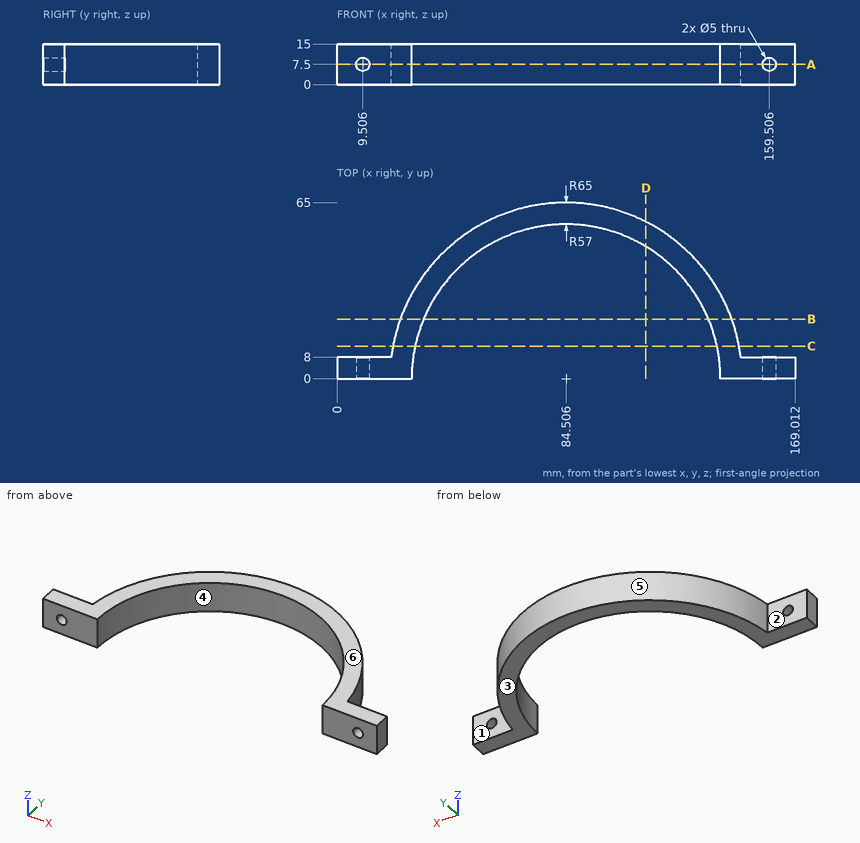
The drawing under review shows one solid part. Ordinate dimensions are in mm from its lowest x, y, z. A direction names the side the tool comes from. Round coordinates to 2 decimals unless told otherwise and drop trailing zeros. Write each loop counter-clockwise with the first axis right and the second up, starting at its lowest first coordinate (ties: lowest second). Pieces come first, ordered by that corner, then holes. Notation, with made-up numbers: (81.25, 50) - (93.25, 50) arc R21 ccw to (93.25, 54) - close; hole circle Ø7 at (-33.5, 86). An arc over 180 degrees is marked (long way). Use one line per item in the form item = value.
Q1. For line 1 (X direction, y = 47, z = 8.75) (1 decimal); line 2 (Y direction, x = 14, z = 10); line 3 (Y direction, x = 135, z = 5) (1 decimal), list the stretches that pass through material, from the lowest coordinate up. Write a range as [from, to].
Answer key:
line_1 = [39.6, 52.3], [116.8, 129.4]
line_2 = [0, 8]
line_3 = [26.4, 40.9]
Q2. Consider section A-A (z = 7.5). State the section outline as (x, y) points.
Answer key:
outline = (0, 0) - (7.01, 0) - (7.01, 8) - (0, 8) - close; (12.01, 0) - (27.51, 0) arc R57 cw to (141.51, 0) - (157.01, 0) - (157.01, 8) - (149.01, 8) arc R65 ccw to (20, 8) - (12.01, 8) - close; (162.01, 0) - (169.01, 0) - (169.01, 8) - (162.01, 8) - close
Q3. Insertion check: pin 1 Ø2 at (x, z) = (90.5, 10) entering from +Y; pin 2 Ø7.5 at (x, z) = (163.5, 9) entering from +Y; pin 3 Ø1.5 at (x, z) = (127, 8.5) entering from +Y (1 decimal). Each pin has a flat end and moves straight along its axis. Give the tip position at first contact, or say it passes through.
Answer key:
pin_1 = 64.81
pin_2 = 8
pin_3 = 49.8
Q4. Consider section B-B (y = 22). State the section outline as (x, z) points.
Answer key:
outline = (23.34, 0) - (31.92, 0) - (31.92, 15) - (23.34, 15) - close; (137.09, 0) - (145.67, 0) - (145.67, 15) - (137.09, 15) - close
Q5. Consider section C-C (y = 12). State the section outline as (x, z) points.
Answer key:
outline = (20.62, 0) - (28.78, 0) - (28.78, 15) - (20.62, 15) - close; (140.23, 0) - (148.39, 0) - (148.39, 15) - (140.23, 15) - close
Q6. Tool access review of the marked faces 1, 2 and 3: name each direction out of +Z, -Z, +X, -X, +Y, -Y from which nothing blocks a thin tool from reaching the whole face with its end or side.
Answer key:
face_1 = +Z, -Z, +X, +Y
face_2 = +Z, -Z, -X, +Y
face_3 = -Z, +X, -X, +Y, -Y
Q7. Draft analysis for pull direction X (two halves, no side actions). For the marked faces 4, 5 and 6, state which applies: +X half, -X half, draft (parallel to the pull), parting line (faces both ways), or undercut.
Answer key:
face_4 = undercut
face_5 = parting line
face_6 = draft
Q8. Consider section D-D (x = 114). State the section outline as (y, z) points.
Answer key:
outline = (48.78, 0) - (57.92, 0) - (57.92, 15) - (48.78, 15) - close
